For this review, take the finished solid that the model builds, in its own axes (mm). Round coordinates to 2 decimals unless told otherwise and drop trailing zeros. Order: outer loops, then holes, each group sorted by start corner. A loop starts at its lowest first (then second) coordinate and runs counter-clockwise, first axis right, second up.
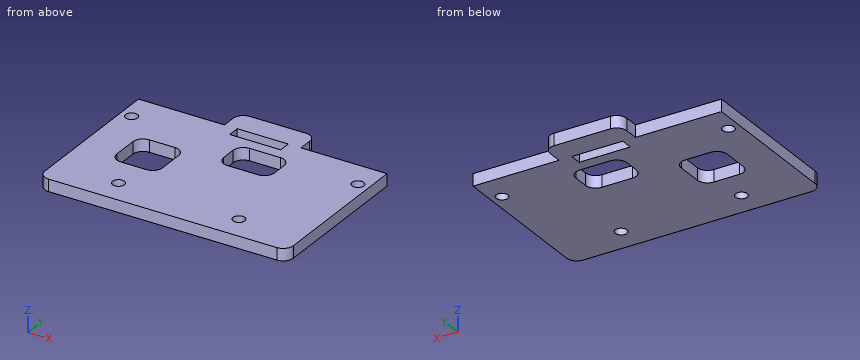
```python
from build123d import *

# Parameters (mm, degrees)
SKETCH1_W                   = 61.88
SKETCH1_H                   = 45.878000096
BOSS_EXTRUDE1_DEPTH         = 3
F_32_0_116_DIAMETER_HOLE1_D = 2.9464
FILLET1_R                   = 2.54
SKETCH6_W                   = 12.7
SKETCH6_H                   = 3
CUT_EXTRUDE1_DEPTH          = 3
SKETCH7_W                   = 12.7
SKETCH7_H                   = 8.89
SKETCH7_W_2                 = 11.43
SKETCH7_H_2                 = 11.43
CUT_EXTRUDE2_DEPTH          = 78.090370947
FILLET2_R                   = 2.54
SKETCH9_W                   = 21.4122
SKETCH9_H                   = 6.000000096
SKETCH9_W_2                 = 21.4178
CUT_EXTRUDE3_DEPTH          = 78.090370947
FILLET4_R                   = 2.54


with BuildPart() as part:
    # Sketch1 → Boss-Extrude1 (new body)
    with BuildSketch(Plane.XY):
        with Locations((30.94, 22.939000048)):
            Rectangle(SKETCH1_W, SKETCH1_H)
    extrude(amount=BOSS_EXTRUDE1_DEPTH)

    # #32 (0.116) Diameter Hole1 (through all)
    with Locations(Plane.XY.offset(3)):
        with Locations((15.954, 6.373999952), (45.926, 6.373999952), (59.11, 32.7152), (2.77, 32.7152)):
            Hole(F_32_0_116_DIAMETER_HOLE1_D / 2)

    # Fillet1
    fillet1_edges = [part.edges().sort_by_distance(p)[0] for p in [
        (61.88, 0, 1.5),
        (0, 0, 1.5),
    ]]
    fillet(fillet1_edges, radius=FILLET1_R)

    # Sketch6 → Cut-Extrude1 (cut)
    with BuildSketch(Plane(origin=(0, 0, 0), x_dir=(-1, 0, 0), z_dir=(0, 0, -1))):
        with Locations((-30.9428, 38.378)):
            Rectangle(SKETCH6_W, SKETCH6_H)
    extrude(amount=-CUT_EXTRUDE1_DEPTH, mode=Mode.SUBTRACT)

    # Sketch7 → Cut-Extrude2 (cut, through all)
    with BuildSketch(Plane(origin=(0, 0, 0), x_dir=(-1, 0, 0), z_dir=(0, 0, -1))):
        with Locations((-35.21, 29.495000096)):
            Rectangle(SKETCH7_W, SKETCH7_H)
        with Locations((-14.605, 20.193)):
            Rectangle(SKETCH7_W_2, SKETCH7_H_2)
    extrude(amount=-CUT_EXTRUDE2_DEPTH, mode=Mode.SUBTRACT)

    # Fillet2
    fillet2_edges = [part.edges().sort_by_distance(p)[0] for p in [
        (41.56, 25.050000096, 1.5),
        (41.56, 33.940000096, 1.5),
        (28.86, 33.940000096, 1.5),
        (28.86, 25.050000096, 1.5),
        (20.32, 14.478, 1.5),
        (20.32, 25.908, 1.5),
        (8.89, 25.908, 1.5),
        (8.89, 14.478, 1.5),
    ]]
    fillet(fillet2_edges, radius=FILLET2_R)

    # Sketch9 → Cut-Extrude3 (cut, through all)
    with BuildSketch(Plane(origin=(0, 0, 0), x_dir=(-1, 0, 0), z_dir=(0, 0, -1))):
        with Locations((-51.1739, 42.878000048)):
            Rectangle(SKETCH9_W, SKETCH9_H)
        with Locations((-10.7089, 42.878000048)):
            Rectangle(SKETCH9_W_2, SKETCH9_H)
    extrude(amount=-CUT_EXTRUDE3_DEPTH, mode=Mode.SUBTRACT)

    # Fillet4
    fillet4_edges = [part.edges().sort_by_distance(p)[0] for p in [
        (40.4678, 45.878000096, 1.5),
        (21.4178, 45.878000096, 1.5),
    ]]
    fillet(fillet4_edges, radius=FILLET4_R)


solid = part.part
```
Q1. Take a section at B-B, the plane y = 22. State the section outline as (x, z) points.
Q2. Wall thickness on line 1 (Y direction, x = 2.77, z = 1.4); line 2 (Y direction, x = 29.5, z = 1.3); line 3 (X direction, y = 32, z = 2.75): over which ranges is each line inside the solid? List them lowest first.
Q3. Take a section at A-A, the plane x = 19. State the section outline as (y, z) points.
Q4. Clearance check with flat-ended pins moving along their axes: pin 1 (1.5 mm diameter, centred on y = 41.5, z = 1.5, fed in from +X); pin 2 (2.5 mm diameter, centred on x = 2.77, y = 32.72, fed in from +Z). State where each tip first meets the part, or that it passes through.
Q5. Take a section at C-C, the plane z = 0.55. Count the separate pieces of the cut face and the enclosed holes in it, plus the area to 3 significant figures.
Q6. Take a section at D-D, the plane x = 43. State the section outline as (y, z) points.
Working result:
1. outline: (0, 0) - (8.89, 0) - (8.89, 3) - (0, 3) - close; (20.32, 0) - (61.88, 0) - (61.88, 3) - (20.32, 3) - close
2. line 1: y = 0 to 31.24, 34.19 to 39.88
2. line 2: y = 0 to 25.9, 33.09 to 36.88, 39.88 to 45.88
2. line 3: x = 0 to 1.48, 4.06 to 28.93, 41.49 to 57.82, 60.4 to 61.88
3. outline: (0, 0) - (14.79, 0) - (14.79, 3) - (0, 3) - close; (25.6, 0) - (39.88, 0) - (39.88, 3) - (25.6, 3) - close
4. pin 1: stops at x = 40.47
4. pin 2: passes through
5. separate pieces: 1
5. enclosed holes: 7
5. area: 2,280 mm2
6. outline: (0, 0) - (39.88, 0) - (39.88, 3) - (0, 3) - close
